Part model, mm, in its own coordinate system. A direction names the side the tool comes from. Give positions to 0.01 mm unless a question says otherwise; leave off trailing zeros. Write each loop counter-clockwise with the first axis right and the second up, starting at its lowest first coordinate (ties: lowest second). Pieces come first, ordered by that corner, then holes. Notation, with made-up numbers: (-18.5, 80) - (26.5, 80) arc R35 cw to (26.5, 116) - close; hole circle Ø1 at (62, 56). An arc over 180 degrees is marked (long way). Answer in a Markdown table with one row per item. Add a question column.
1. Band-saw the part on A-A on z = 0. Write the cut outline in (x, y), plus the area to 3 significant figures.
2. Probe line 1 along Y through (x, z) = (51, -3.5); line 2 along X through (y, z) = (30, -50); line 3 along Z through (x, y) = (122, 50.5). List the from-to ranges inside material, lowest first.
3. Which spindle directions (+Z, -Z, +X, -X, +Y, -Y) get a long thin tool onto all of the face, cutting with end or side? Do faces 1 (the cylindrical face through (126.298, -15.43, -60.903)), 2 (the flat face through (0, 1, -1)), 3 (the flat face through (124, -16, 66)), 4 (the flat face through (50, 50, -5)), 5 (the conical face through (123.95, -71.185, -1.351)). Say none if no direction does.
4. Pull direction Z, two halves, no side cores. Call faces 6 (the flat face through (126, 16, -66)), 7 (the cylindrical face through (216.22, -0.35, 70.96)), 8 (the conical face through (0.19, -46.07, -10.23)): released by +Z, released by -Z, zero draft, split by the parting line, or undercut.
5. Drop flat-ended pins along their axis: pin 1 Ø16.5 at (x, z) = (125, -69) entering from -Y; pin 2 Ø5 at (x, z) = (53.5, 28) entering from +Y; pin 3 Ø6 at (x, z) = (103, 7.5) entering from +Y; pin 4 Ø12 at (y, z) = (31, 22.5) entering from -X. Give the stop position or say it passes through.
6. Band-saw the part on B-B on y = 0. Write the cut outline in (x, z).
```python
from build123d import *

# Parameters (mm, degrees)
F4_DEPTH = 11
F5_R     = 5
F7_SIZE  = 3
F8_R     = 2


# Not quite as in the source:
# - a pattern or mirror of a feature is missing from the dataset's text; its kind, count and spacing are read off the source's solid


with BuildPart() as f1:
    # F0 (on Front) → F1 (revolve)
    with BuildSketch(Plane.XZ):
        Polygon((0, 50), (0, 0), (227, 0), (227, 75), (200, 75), (50, 67.5), (50, 50), align=None)
    revolve(axis=Axis((113.5, 0, 0), (-1, 0, 0)))

    # F3 (on line) → F4 (cut)
    with BuildSketch(Plane(origin=(-3.2418952618, 0, 64.8379052369), x_dir=(0.9987523389, 0, 0.0499376169), z_dir=(-0.0499376169, 0, 0.9987523389))):
        with BuildLine():
            Line((0, 16), (0, -16))
            Line((0, -16), (203.4957890464, -16))
            ThreePointArc((203.4957890464, -16), (219.4957890464, 0), (203.4957890464, 16))
            Line((203.4957890464, 16), (0, 16))
        make_face()
    f4 = extrude(amount=-F4_DEPTH, mode=Mode.SUBTRACT)

    # F4_copies: F4 across plane
    add(f4.mirror(Plane(origin=(0, 0, -1e-06), x_dir=(-1, 0, 0), z_dir=(0, 0, -1))), mode=Mode.SUBTRACT)

    # F5 (on Front) → F6 (revolve, cut)
    with BuildSketch(Plane.XZ):
        with Locations((201.5, 79.8)):
            Circle(F5_R)
    revolve(axis=Axis((113.5, 0, 0), (-1, 0, 0)), mode=Mode.SUBTRACT)

    # F7
    f7_edges = [f1.edges().sort_by_distance(p)[0] for p in [
        (0, 0, -50),
    ]]
    chamfer(f7_edges, length=F7_SIZE)

    # F8
    f8_edges = [f1.edges().sort_by_distance(p)[0] for p in [
        (125.274657, 16, 60.249991),
        (216.529351, 0, 64.812726),
        (125.274657, -16, 60.249991),
        (125.274657, -16, -60.249993),
        (216.529351, 0, -64.812728),
        (125.274657, 16, -60.249993),
    ]]
    fillet(f8_edges, radius=F8_R)


solid = f1.part
```
Values:
| question | item | result |
|---|---|---|
| 1 | outline | (0, -47) - (3, -50) - (50, -50) - (50, -67.5) - (200, -75) - (200.1, -75) arc R5 cw to (202.9, -75) - (227, -75) - (227, 75) - (202.9, 75) arc R5 cw to (200.1, 75) - (200, 75) - (50, 67.5) - (50, 50) - (3, 50) - (0, 47) - close |
| 1 | area | 30,400 mm² |
| 2 | line 1 | y = -67.46 to 67.46 |
| 2 | line 2 | x = 50 to 227 |
| 2 | line 3 | z = -50.05 to 50.05 |
| 3 | face 1 | -Z, -X |
| 3 | face 2 | +Z, -Z, -X, +Y, -Y |
| 3 | face 3 | +Z, -X |
| 3 | face 4 | -X |
| 3 | face 5 | -X, -Y |
| 4 | face 6 | zero draft |
| 4 | face 7 | undercut |
| 4 | face 8 | split by the parting line |
| 5 | pin 1 | stops at y = -37.25 |
| 5 | pin 2 | stops at y = 62.7 |
| 5 | pin 3 | stops at y = 70.05 |
| 5 | pin 4 | stops at x = 0 |
| 6 | outline | (0, -47) - (3, -50) - (50, -50) - (50, -56.49) - (214.53, -64.71) arc R2 cw to (216.43, -66.81) - (216.02, -75) - (227, -75) - (227, 75) - (216.02, 75) - (216.43, 66.81) arc R2 cw to (214.53, 64.71) - (50, 56.49) - (50, 50) - (3, 50) - (0, 47) - close |
